Here's how the part is built. I have some questions about the finished solid (model axes, mm). Face numbers are marked on the shaded views. A direction names the side the tool comes from. Coordinates: 2 decimals unless noted, no trailing zeros. Loops run counter-clockwise (first coordinate to the right, second up) from the corner with the lowest first, then second, coordinate; pieces in that order, holes last.
from build123d import *

# Parameters (mm, degrees)
F0_R     = 3.9
F1_DEPTH = 25
F0_R_2   = 15
F2_DEPTH = 5
F3_W     = 2
F3_H     = 2


with BuildPart() as f1:
    # F0 (on Top) → F1 (new body)
    with BuildSketch(Plane.XY):
        Circle(F0_R)
    extrude(amount=F1_DEPTH)

    # F0 (on Top) → F2 (join)
    with BuildSketch(Plane.XY):
        Circle(F0_R_2)
        Circle(F0_R, mode=Mode.SUBTRACT)
    extrude(amount=F2_DEPTH)

    # F3 (on Right) → F4 (revolve, cut)
    with BuildSketch(Plane.YZ):
        with Locations((15, 2.5)):
            Rectangle(F3_W, F3_H)
    revolve(axis=Axis((0, 0, 5), (0, 0, 1)), mode=Mode.SUBTRACT)


solid = f1.part
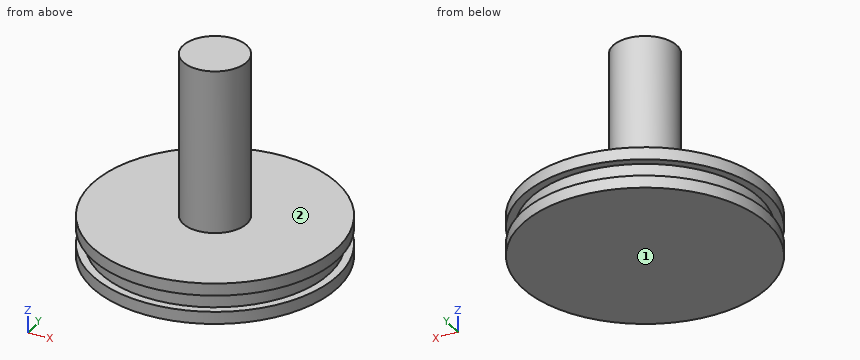
Q1. Suppose I cut it at A-A on y = 0. Write out the boundary of the cut face in (x, z), and give its area (3 significant figures).
Q2. Will these pins go through, and if not, where does the flat tip stop? P1, Ø4, axis at y = -0.5, z = 14, coming from the +X side; P2, Ø1.5, axis at y = -1.5, z = 18.5, coming from the -X side; P3, Ø4, axis at x = -3, z = 12, coming from the +Y side.
Q3. Please list where these lines run through material, in increasing order: probe 1 along Z at (x, y) = (-7.5, -12.5); probe 2 along Z at (x, y) = (-2.75, 5.5); probe 3 along X at (y, z) = (3.5, 17.5).
Q4. Suppose I cut it at C-C on z = 21.5. Write out the boundary of the cut face in (x, y).
Q5. Suppose I cut it at D-D on x = -12. Write out the boundary of the cut face in (y, z), and give its area (3 significant figures).
Q6. For the marked faces 1 and 2, which set-ups out of +Z, -Z, +X, -X, +Y, -Y let a thin tool reach every point of the face, with its end or its side?
Check values:
1. outline: (-15, 0) - (15, 0) - (15, 1.5) - (14, 1.5) - (14, 3.5) - (15, 3.5) - (15, 5) - (3.9, 5) - (3.9, 25) - (-3.9, 25) - (-3.9, 5) - (-15, 5) - (-15, 3.5) - (-14, 3.5) - (-14, 1.5) - (-15, 1.5) - close
1. area: 302 mm2
2. P1: stops at x = 3.9
2. P2: stops at x = -3.83
2. P3: stops at y = 3.77
3. probe 1: z = 0 to 1.5, 3.5 to 5
3. probe 2: z = 0 to 5
3. probe 3: x = -1.72 to 1.72
4. outline: circle Ø7.8 at (0, 0)
5. outline: (-9, 0) - (9, 0) - (9, 1.5) - (7.21, 1.5) - (7.21, 3.5) - (9, 3.5) - (9, 5) - (-9, 5) - (-9, 3.5) - (-7.21, 3.5) - (-7.21, 1.5) - (-9, 1.5) - close
5. area: 82.8 mm2
6. face 1: -Z, +X, -X, +Y, -Y
6. face 2: +Z
